from build123d import *
from OCP.BRepFilletAPI import BRepFilletAPI_MakeChamfer

# Parameters (mm, degrees)
BOSS_EXTRUDE1_DEPTH = 18
SKETCH2_R           = 1.5
BOSS_EXTRUDE2_DEPTH = 20
SKETCH3_W           = 8
SKETCH3_H           = 7
BOSS_EXTRUDE3_DEPTH = 5
SKETCH4_R           = 1.5
CUT_EXTRUDE1_DEPTH  = 10
CHAMFER1_SIZE       = 16
CHAMFER1_SIZE2      = 7.46092253
FILLET3_R           = 2


with BuildPart() as part:
    # Sketch1 → Boss-Extrude1 (new body)
    with BuildSketch(Plane(origin=(0, 0, 0), x_dir=(1, 0, 0), z_dir=(0, 1, 0))):
        with BuildLine():
            Line((0, 0), (-39, 0))
            ThreePointArc((-39, 0), (-54.5, 15.5), (-39, 31))
            Line((-39, 31), (0, 31))
            ThreePointArc((0, 31), (15.5, 15.5), (0, 0))
        make_face()
    extrude(amount=BOSS_EXTRUDE1_DEPTH)

    # Sketch2 → Boss-Extrude2 (add)
    with BuildSketch(Plane(origin=(0, 18, 0), x_dir=(1, 0, 0), z_dir=(0, 1, 0))):
        with Locations(Location((-6.5, 12, 0), (0, 0, 90))):
            Circle(SKETCH2_R)
    extrude(amount=BOSS_EXTRUDE2_DEPTH)

    # Sketch3 → Boss-Extrude3 (add)
    with BuildSketch(Plane(origin=(0, 18, 0), x_dir=(1, 0, 0), z_dir=(0, 1, 0))):
        with Locations((-28.5, 15.5)):
            Rectangle(SKETCH3_W, SKETCH3_H)
    extrude(amount=BOSS_EXTRUDE3_DEPTH)

    # Sketch4 → Cut-Extrude1 (cut)
    with BuildSketch(Plane.ZY.offset(32.5)):
        with Locations((-15.5, 20)):
            Circle(SKETCH4_R)
        with BuildLine():
            Line((-19, 19.5), (-19, 26.550877956))
            Line((-19, 26.550877956), (-12, 26.550877956))
            Line((-12, 26.550877956), (-12, 19.5))
            ThreePointArc((-12, 19.5), (-15.5, 23), (-19, 19.5))
        make_face()
    extrude(amount=-CUT_EXTRUDE1_DEPTH, mode=Mode.SUBTRACT)

    # Chamfer1: one chamfer whose edges measure the first distance from different faces: ONE call of the kernel's chamfer builder (chamfer() names one face for all edges)
    chamfer1_edges_1 = [part.edges().sort_by_distance(p)[0] for p in [
        (-54.5, 18, -15.5),
    ]]
    chamfer1_side_1 = [part.faces().sort_by_distance(p)[0] for p in [
        (-54.5, 9, -15.5),
    ]]
    chamfer1_edges_2 = [part.edges().sort_by_distance(p)[0] for p in [
        (-19.5, 18, 0),
    ]]
    chamfer1_side_2 = [part.faces().sort_by_distance(p)[0] for p in [
        (-19.5, 9, 0),
    ]]
    chamfer1_edges_3 = [part.edges().sort_by_distance(p)[0] for p in [
        (15.5, 18, -15.5),
    ]]
    chamfer1_side_3 = [part.faces().sort_by_distance(p)[0] for p in [
        (15.5, 9, -15.5),
    ]]
    chamfer1_edges_4 = [part.edges().sort_by_distance(p)[0] for p in [
        (-19.5, 18, -31),
    ]]
    chamfer1_side_4 = [part.faces().sort_by_distance(p)[0] for p in [
        (-19.5, 9, -31),
    ]]
    chamfer1 = BRepFilletAPI_MakeChamfer(part.part.solid().wrapped)
    for e in chamfer1_edges_1:
        chamfer1.Add(CHAMFER1_SIZE, CHAMFER1_SIZE2, e.wrapped, chamfer1_side_1[0].wrapped)  # the first distance lies on this face
    for e in chamfer1_edges_2:
        chamfer1.Add(CHAMFER1_SIZE, CHAMFER1_SIZE2, e.wrapped, chamfer1_side_2[0].wrapped)  # the first distance lies on this face
    for e in chamfer1_edges_3:
        chamfer1.Add(CHAMFER1_SIZE, CHAMFER1_SIZE2, e.wrapped, chamfer1_side_3[0].wrapped)  # the first distance lies on this face
    for e in chamfer1_edges_4:
        chamfer1.Add(CHAMFER1_SIZE, CHAMFER1_SIZE2, e.wrapped, chamfer1_side_4[0].wrapped)  # the first distance lies on this face
    add(Compound.cast(chamfer1.Shape()), mode=Mode.REPLACE)

    # Fillet3
    fillet3_edges = [part.edges().sort_by_distance(p)[0] for p in [
        (-19.5, 18, -23.53907747),
        (-47.03907747, 18, -15.5),
        (8.03907747, 18, -15.5),
        (-19.5, 18, -7.46092253),
        (-19.5, 2, 0),
        (15.5, 2, -15.5),
        (-54.5, 2, -15.5),
        (-19.5, 2, -31),
    ]]
    fillet(fillet3_edges, radius=FILLET3_R)


solid = part.part
Could you check a few things on this model? Use its own coordinates, in mm. A direction names the side the tool comes from. Round coordinates to 2 decimals unless told otherwise and drop trailing zeros. Write each loop counter-clockwise with the first axis right and the second up, starting at its lowest first coordinate (ties: lowest second). Pieces come first, ordered by that corner, then holes. Notation, with made-up numbers: (-38.75, 35.5) -> (-32.75, 35.5) arc R17 cw to (-32.75, 42.5) -> close; hole circle Ø8 at (-9.5, 43.25). An arc over 180 degrees is marked (long way). Use a Markdown table: item, result.
1. Please list where these lines run through material, in increasing order: probe 1 along Y at (x, z) = (-29, -15.5); probe 2 along Y at (x, z) = (-30, -15); probe 3 along Y at (x, z) = (-36.5, -20).
Answer key:
| item | result |
|---|---|
| probe 1 | y = 0 to 18.5, 21.5 to 23 |
| probe 2 | y = 0 to 18.59, 21.41 to 22.96 |
| probe 3 | y = 0 to 18 |
2. If we section it at B-B (y = 8.5): List the corners of the cut face in (x, z) for me.
Answer key:
| item | result |
|---|---|
| outline | (-39, -27.97) -> (0, -27.97) arc R12.47 ccw to (0, -3.03) -> (-39, -3.03) arc R12.47 ccw to start |
3. For pin 1 Ø2.5 at (y, z) = (20.5, -16.5) entering from -X; pin 2 Ø5 at (x, z) = (-16, -7) entering from +Y; pin 3 Ø4 at (y, z) = (18, -20.5) entering from -X, each with a flat end and sliding along its axis, tell me the tip position at first contact or that it passes through.
Answer key:
| item | result |
|---|---|
| pin 1 | stops at x = -32.5 |
| pin 2 | stops at y = 18 |
| pin 3 | stops at x = -46.93 |
4. If we section it at A-A (x = -10): List the corners of the cut face in (y, z) for me, then the cut area to 3 significant figures.
Answer key:
| item | result |
|---|---|
| outline | (0, -31) -> (1.56, -31) arc R2 ccw to (2.4, -30.81) -> (16.85, -24.08) arc R2 ccw to (18, -22.26) -> (18, -8.74) arc R2 ccw to (16.85, -6.92) -> (2.4, -0.19) arc R2 ccw to (1.56, 0) -> (0, 0) -> close |
| area | 438 mm^2 |
5. We'd pull the mould along X, two halves only. Please class faces 5 (the face through (-24.5, 22, -15)), 6 (the face through (-19.77, 9.72, -27.4)), 7 (the face through (-32.5, 22, -15)), 8 (the face through (15.496, 0.767, -15.841)): +X half, -X half, draft (parallel to the pull), parting line (faces both ways), or undercut.
Answer key:
| item | result |
|---|---|
| face 5 | undercut |
| face 6 | draft |
| face 7 | -X half |
| face 8 | +X half |
6. Which directions (+Z, -Z, +X, -X, +Y, -Y) give clear straight access to the entire face, cutting with the end or side of a thin tool? Please do faces 1 (the face through (-19, 0, -16)), 2 (the face through (-29, 19, -19)), 3 (the face through (-28.6, 23, -15.4)), 4 (the face through (-5.6, 27.9, -10.8)).
Answer key:
| item | result |
|---|---|
| face 1 | +Z, -Z, +X, -X, -Y |
| face 2 | -Z, +X, -X, +Y |
| face 3 | -X, +Y |
| face 4 | +Y |
